Read the model definition and answer for the solid it produces. Units are mm, in the model's axes. Coordinates: 2 decimals unless noted, no trailing zeros. Write each loop counter-clockwise with the first axis right and the second up, starting at its lowest first coordinate (ties: lowest second). Pieces come first, ordered by that corner, then holes. Notation, with made-up numbers: (49, 34.25) -> (60, 34.25) arc R15 cw to (60, 59.25) -> close; hole circle Ø10 at (50, -13.75). An arc over 180 degrees is marked (long way). Write item = value, one per line. Start each with the question number.
1) Section B-B (y = -1.45) is taken. Determine the outline of the cut face in (x, z).
2) Find the intervals of material crossed by line 1 along X through (y, z) = (-0.7, 34); line 2 along X through (y, z) = (-0.6, -26); line 3 along Z through (x, y) = (-135.5, -2.8), in increasing order. Write a range as from..to.
3) Section C-C (x = -29) is taken. Determine the outline of the cut face in (y, z), plus the area to 3 significant figures.
4) Section A-A (z = 63) is taken. Determine the outline of the cut face in (x, y).
from build123d import *

# Parameters (mm, degrees)
F1_DEPTH = 3
F2_R     = 10


with BuildPart() as f1:
    # F0 (on Front) → F1 (new body)
    with BuildSketch(Plane.XZ):
        Polygon((-225, 75), (-225, -75), (225, -75), (225, 75), (-25, 75), (-25, -35), (-55, -35), (-55, 75), (-95, 75), (-95, -35), (-145, -35), (-145, 75), align=None)
    extrude(amount=F1_DEPTH)

    # F2
    f2_edges = [f1.edges().sort_by_distance(p)[0] for p in [
        (-145, -1.5, -35),
        (-95, -1.5, -35),
        (-25, -1.5, -35),
        (-55, -1.5, -35),
    ]]
    fillet(f2_edges, radius=F2_R)


solid = f1.part
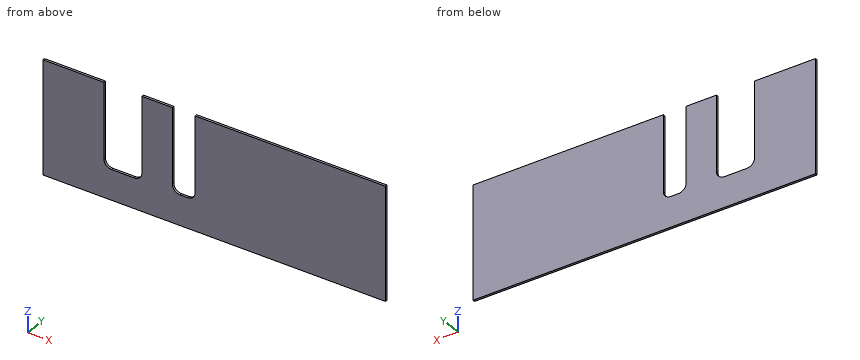
Answer key:
q1.outline = (-225, -75) -> (225, -75) -> (225, 75) -> (-25, 75) -> (-25, -25) arc R10 cw to (-35, -35) -> (-45, -35) arc R10 cw to (-55, -25) -> (-55, 75) -> (-95, 75) -> (-95, -25) arc R10 cw to (-105, -35) -> (-135, -35) arc R10 cw to (-145, -25) -> (-145, 75) -> (-225, 75) -> close
q2.line_1 = -225..-145, -95..-55, -25..225
q2.line_2 = -225..-144.95, -95.05..-54.95, -25.05..225
q2.line_3 = -75..-34.99
q3.outline = (-3, -75) -> (0, -75) -> (0, -33) -> (-3, -33) -> close
q3.area = 126 mm^2
q4.outline = (-225, -3) -> (-145, -3) -> (-145, 0) -> (-225, 0) -> close; (-95, -3) -> (-55, -3) -> (-55, 0) -> (-95, 0) -> close; (-25, -3) -> (225, -3) -> (225, 0) -> (-25, 0) -> close
